```python
from build123d import *

# Parameters (mm, degrees)
BASENUTSKE_R   = 7
BASENUT_DEPTH  = 16
FLANGEFILLET_R = 0.96


with BuildPart() as part:
    # BaseNutSke → BaseNut (new body)
    with BuildSketch(Plane.XY):
        Polygon((12, 6.92820323), (12, -6.92820323), (0, -13.856406461), (-12, -6.92820323), (-12, 6.92820323), (0, 13.856406461), align=None)
        Circle(BASENUTSKE_R, mode=Mode.SUBTRACT)
    extrude(amount=-BASENUT_DEPTH)

    # Sketch6 → Flange (revolve)
    with BuildSketch(Plane(origin=(0, 0, 0), x_dir=(0, 0, -1), z_dir=(1, 0, 0)), mode=Mode.PRIVATE) as flange_sk:
        with BuildLine():
            Line((10.165622253, 7), (13.6, 16.435875309))
            ThreePointArc((13.6, 16.435875309), (14.977547085, 17.231202489), (16, 16.012690555))
            Line((16, 16.012690555), (16, 7))
            Line((16, 7), (10.165622253, 7))
        make_face()
    revolve(flange_sk.sketch.rotate(Axis((0, 0, 0), (0, 0, -1)), 90), axis=Axis((0, 0, 0), (0, 0, -1)))

    # Sketch3 → Double-Chamfer (revolve, cut)
    with BuildSketch(Plane(origin=(0, 0, 0), x_dir=(0, 0, -1), z_dir=(1, 0, 0)), mode=Mode.PRIVATE) as double_chamfer_sk:
        Polygon((1.6, 26.556406461), (-12.7, 26.556406461), (-12.7, 12), (0, 12), (1.6, 13.856406461), align=None)
    revolve(double_chamfer_sk.sketch.rotate(Axis((0, 0, 0), (0, 0, -1)), 90), axis=Axis((0, 0, 0), (0, 0, -1)), mode=Mode.SUBTRACT)

    # FlangeFillet
    flangefillet_edges = [part.edges().sort_by_distance(p)[0] for p in [
        (12, -3.479213152, -12.16534592),
        (12, 3.479213152, -12.16534592),
        (6, -10.392304845, -11.985473425),
        (6, 10.392304845, -11.985473425),
        (-6, 10.392304845, -11.985473425),
        (-12, 0, -11.985473425),
        (-6, -10.392304845, -11.985473425),
    ]]
    fillet(flangefillet_edges, radius=FLANGEFILLET_R)

    # Sketch5 (on Right Plane) → EndChamfer (revolve, cut)
    with BuildSketch(Plane(origin=(0, 0, 0), x_dir=(0, 0, -1), z_dir=(1, 0, 0)), mode=Mode.PRIVATE) as endchamfer_sk:
        Polygon((15.9746, 8), (15.204371708, 6.9), (16.0254, 6.9), (16.0254, 8), align=None)
        Polygon((-0.0508, 8), (0, 8), (0.770228292, 6.9), (-0.0508, 6.9), align=None)
    revolve(endchamfer_sk.sketch.rotate(Axis((0, 0, -25.037505729), (0, 0, -1)), 90), axis=Axis((0, 0, -25.037505729), (0, 0, -1)), mode=Mode.SUBTRACT)


solid = part.part
```
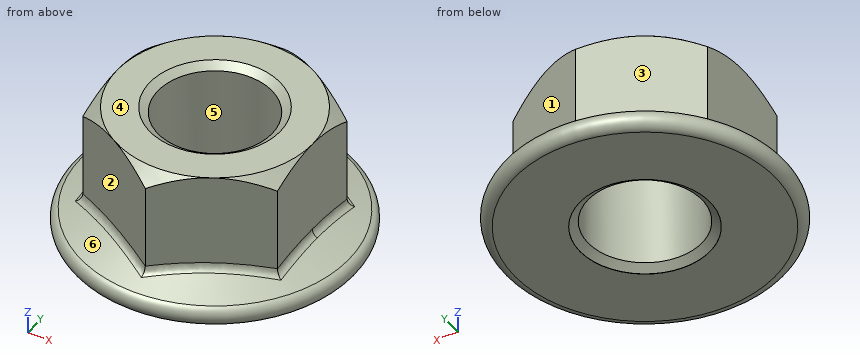
Read the model definition and answer for the solid it produces. Units are mm, in the model's axes. Face numbers are marked on the shaded views. A direction names the side the tool comes from. Round coordinates to 2 decimals unless told otherwise and drop trailing zeros. Write each loop counter-clockwise with the first axis right and the second up, starting at its lowest first coordinate (ties: lowest second). Pieces come first, ordered by that corner, then holes. Notation, with made-up numbers: (6, 63.5) - (63, 63.5) arc R26 ccw to (63, 95.5) - close; hole circle Ø9 at (74, -30.5). An arc over 180 degrees is marked (long way). Use CSV: the item, a comma, the result in double quotes.
Q1. A tool of negligible diameter and unlimited length cuts with its end or side. For the marked faces 1, 2 and 3, from which of +Z, -Z, +X, -X, +Y, -Y can it reach the whole face along a straight path? Write none if from no direction.
Values:
face 1,"+Z, +X, +Y"
face 2,"+Z, -X, -Y"
face 3,"+Z, -X, +Y"
Q2. Find section B-B, the plane z = -14.5. Write down the section's boundary in (x, y), then the cut area to 3 significant figures.
Values:
outline,"circle Ø34.44 at (0, 0); hole circle Ø14 at (0, 0)"
area,"778 mm²"
Q3. Find section A-A, the plane z = -9.5. Write down the section's boundary in (x, y).
Values:
outline,"(-12, -6.93) - (0, -13.86) - (12, -6.93) - (12, 6.93) - (0, 13.86) - (-12, 6.93) - close; hole circle Ø14 at (0, 0)"
Q4. Each of these flat-tipped pins is pushed along its axis until it touches: pin 1 Ø1 at (x, y) = (-13, -11) entering from -Z; pin 2 Ø14.5 at (x, y) = (0, 0) entering from +Z; pin 3 Ø3 at (x, z) = (0.5, -7) entering from -Y; pin 4 Ø12.5 at (x, y) = (0, 0) entering from -Z. Where does it stop, or does it pass through?
Values:
pin 1,"stops at z = -15.89"
pin 2,"stops at z = -0.53"
pin 3,"stops at y = -13.86"
pin 4,"passes through"
Q5. Straight lines are drawn through the part: line 1 along Y through (x, z) = (0, -4); line 2 along Y through (x, z) = (-1, -3.75); line 3 along X through (y, z) = (-3, -3.5). For each, find the intervals that lie inside material, in ascending order.
Values:
line 1,"y = -13.86 to -7, 7 to 13.86"
line 2,"y = -13.28 to -6.93, 6.93 to 13.28"
line 3,"x = -12 to -6.32, 6.32 to 12"
Q6. Determine the mould class of the marked faces 4, 5 and 6 for opening direction Y: +Y half, -Y half, draft (parallel to the pull), parting line (faces both ways), or undercut.
Values:
face 4,"draft"
face 5,"undercut"
face 6,"parting line"
